Part model, mm, in its own coordinate system. Round coordinates to 2 decimals unless told otherwise and drop trailing zeros. Order: outer loops, then holes, each group sorted by start corner. A loop starts at its lowest first (then second) coordinate and runs counter-clockwise, first axis right, second up. Notation, with made-up numbers: (40.5, -40) -> (71.5, -40) arc R24 cw to (71.5, -16) -> close; hole circle Ø11 at (13, 22). An arc over 180 degrees is marked (long way). Use CSV: the item, a comma, the result in double quotes.
Autodesk Inventor part; units mm, degrees
ref_plane "YZ Plane" through (0, 0, 0) normal (1, 0, 0) x (0, 1, 0)
ref_plane "XZ Plane" through (0, 0, 0) normal (0, 1, 0) x (-1, 0, 0)
ref_plane "XY Plane" through (0, 0, 0) normal (0, 0, 1) x (1, 0, 0)
sketch "Sketch1" plane through (0, 0, 0) normal (0, 0, 1) x (1, 0, 0)
  circle A0 centre (0, 0) radius 15.24
  dimension "d0" = 30.48
extrude "Extrusion1" add sketch "Sketch1" along normal mid plane 96.52
sketch "Sketch2" plane through (0, 0, 0) normal (1, 0, 0) x (0, 1, 0)
  line L0 (15.24, -48.26) -> (-15.24, -48.26)
  line L1 (-15.24, -48.26) -> (-15.24, 48.26)
  line L2 (-15.24, 48.26) -> (15.24, 48.26)
  line L3 (15.24, 48.26) -> (15.24, -48.26)
  line L4 (-15.24, -48.26) -> (15.24, -48.26)
  line L5 (15.24, 48.26) -> (-15.24, 48.26)
  line L6 (-21.336, 0) -> (21.336, 0)
  line L7 (0, -67.564) -> (0, 67.564)
  circle A0 centre (0, 35.56) radius 3.81
  circle A1 centre (0, -35.56) radius 3.81
  point P0 (0, 0)
  dimension "d3" = 7.62
  dimension "d4" = 7.62
  dimension "d5" = 12.7
  dimension "d6" = 12.7
extrude "Extrusion2" cut sketch "Sketch2" against normal through all both and the other way through all contours A1 L7 | L7 A1 | A0 L7 | L7 A0
chamfer "Chamfer1" distance 1.27 angle 45 2 edges at (-15.24, 0, 48.26) (-15.24, 0, -48.26) measured on face at (9.6385, 11.805, 16.0867)
equation "\"BendRadius\" = Thickness"
equation "\"BendReliefWidth\" = Thickness"
equation "\"BendReliefDepth\" = 0.5 * Thickness"
equation "\"CornerReliefSize\" = 4 * Thickness"
equation "\"MinimumRemnant\" = 2 * Thickness"
equation "\"TransitionRadius\" = BendRadius"
equation "\"JacobiRadiusSize\" = BendRadius"
equation "\"GapSize\" = Thickness"
properties part number "crankshaft pin" material "Stainless Steel"
(1) Cut at D-D, the plane z = -35.56. Give the cut face in (x, y).
Reply:
outline,"(-14.76, -3.81) arc R15.24 ccw to (14.76, -3.81) -> close; (-14.76, 3.81) -> (14.76, 3.81) arc R15.24 ccw to start"
(2) Pull direction Y, two halves, no side cores. Call faces 1 (the face through (0, 0, 48.26)), 2 (the face through (0.213, -0.496, -31.782)), 3 (the face through (14.078, 5.837, -0.658)): released by +Y, released by -Y, zero draft, split by the parting line, or undercut.
Reply:
face 1,"zero draft"
face 2,"undercut"
face 3,"split by the parting line"
(3) Cut at B-B, the plane x = 0. Give the cut face in (y, z), then the cut area to 3 significant figures.
Reply:
outline,"(-15.24, -46.99) -> (-13.97, -48.26) -> (13.97, -48.26) -> (15.24, -46.99) -> (15.24, 46.99) -> (13.97, 48.26) -> (-13.97, 48.26) -> (-15.24, 46.99) -> close; hole circle Ø7.62 at (0, -35.56); hole circle Ø7.62 at (0, 35.56)"
area,"2,850 mm2"
(4) Probe probe 1 along Z at (x, y) = (9.5, 0); probe 2 along Z at (x, y) = (0.5, 3); probe 3 along Y at (x, z) = (-6, 36.5). List the from-to ranges inside material, lowest first. Write a range as [from, to].
Reply:
probe 1,"[-48.26, -39.37], [-31.75, 31.75], [39.37, 48.26]"
probe 2,"[-48.26, -37.91], [-33.21, 33.21], [37.91, 48.26]"
probe 3,"[-14.01, -3.69], [3.69, 14.01]"
(5) Cut at A-A, the plane y = 0. Give the cut face in (x, z).
Reply:
outline,"(-15.24, -46.99) -> (-13.97, -48.26) -> (13.97, -48.26) -> (15.24, -46.99) -> (15.24, -39.37) -> (-15.24, -39.37) -> close; (-15.24, -31.75) -> (15.24, -31.75) -> (15.24, 31.75) -> (-15.24, 31.75) -> close; (-15.24, 39.37) -> (15.24, 39.37) -> (15.24, 46.99) -> (13.97, 48.26) -> (-13.97, 48.26) -> (-15.24, 46.99) -> close"
(6) Cut at C-C, the plane z = -8. Give the cut face in (x, y).
Reply:
outline,"circle Ø30.48 at (0, 0)"
(7) Drop flat-ended pins along their axis: P1, Ø5, axis at y = 10, z = -30, coming from the -X side; P2, Ø1.5, axis at x = 11, z = -29.5, coming from the -Y side; P3, Ø4, axis at x = -4, z = -22, coming from the -Y side; P4, Ø4.5, axis at y = 0, z = -35.56, coming from the +X side. Give the stop position or say it passes through.
Reply:
P1,"x = -13.27"
P2,"y = -11.28"
P3,"y = -15.11"
P4,"through"
